from build123d import *

# Parameters (mm, degrees)
SKETCH_1_R        = 3.75
SKETCH_1_R_2      = 2.75
EXTRUDE_250_DEPTH = 4
EXTRUDE_START     = 4
SKETCH_2_R        = 1.7
SKETCH_2_R_2      = 2.75
EXTRUDE_354_DEPTH = 5


with BuildPart() as part:
    # 草图1 → Extrude 250 (new body)
    with BuildSketch(Plane.XY):
        Polygon((-55, -44), (-49, -50), (49, -50), (55, -44), (55, 44), (49, 50), (-49, 50), (-55, 44), (-55, 10), (12, 10), (12, -10), (-55, -10), align=None)
        with Locations((-14.845, -14.845)):
            Circle(SKETCH_1_R, mode=Mode.SUBTRACT)
        with Locations((-14.845, 14.845)):
            Circle(SKETCH_1_R, mode=Mode.SUBTRACT)
        with Locations((14.845, -14.845)):
            Circle(SKETCH_1_R, mode=Mode.SUBTRACT)
        with Locations((14.845, 14.845)):
            Circle(SKETCH_1_R, mode=Mode.SUBTRACT)
        with Locations((-44, -39)):
            Circle(SKETCH_1_R_2, mode=Mode.SUBTRACT)
        with Locations((-44, 39)):
            Circle(SKETCH_1_R_2, mode=Mode.SUBTRACT)
        with Locations((44, -39)):
            Circle(SKETCH_1_R_2, mode=Mode.SUBTRACT)
        with Locations((44, 39)):
            Circle(SKETCH_1_R_2, mode=Mode.SUBTRACT)
    extrude(amount=EXTRUDE_250_DEPTH)

    # 草图2 → Extrude 354 (add)
    with BuildSketch(Plane.XY.offset(EXTRUDE_START)):
        Polygon((-55, -44), (-49, -50), (49, -50), (55, -44), (55, 44), (49, 50), (-49, 50), (-55, 44), (-55, 10), (12, 10), (12, -10), (-55, -10), align=None)
        with Locations((-14.845, -14.845)):
            Circle(SKETCH_2_R, mode=Mode.SUBTRACT)
        with Locations((-14.845, 14.845)):
            Circle(SKETCH_2_R, mode=Mode.SUBTRACT)
        with Locations((14.845, -14.845)):
            Circle(SKETCH_2_R, mode=Mode.SUBTRACT)
        with Locations((14.845, 14.845)):
            Circle(SKETCH_2_R, mode=Mode.SUBTRACT)
        with Locations((-44, -39)):
            Circle(SKETCH_2_R_2, mode=Mode.SUBTRACT)
        with Locations((-44, 39)):
            Circle(SKETCH_2_R_2, mode=Mode.SUBTRACT)
        with Locations((44, -39)):
            Circle(SKETCH_2_R_2, mode=Mode.SUBTRACT)
        with Locations((44, 39)):
            Circle(SKETCH_2_R_2, mode=Mode.SUBTRACT)
    extrude(amount=EXTRUDE_354_DEPTH)


solid = part.part
For this review, take the finished solid that the model builds, in its own axes (mm). A direction names the side the tool comes from. Coordinates: 2 decimals unless noted, no trailing zeros. Order: outer loops, then holes, each group sorted by start corner. A loop starts at its lowest first (then second) coordinate and runs counter-clockwise, first axis right, second up. Notation, with made-up numbers: (71.5, 25) - (101.5, 25) arc R16 cw to (101.5, 53) - close; hole circle Ø5 at (56, 32.5). An arc over 180 degrees is marked (long way). Answer as CSV lines item,"result". Start each with the question number.
1) Add section B-B (x = 44). State the section outline as (y, z) points.
2) Draft analysis for pull direction Y (two halves, no side actions). For faces 4 (the flat face through (52, -47, 4)), 5 (the flat face through (55, -1, 4)), 6 (the cylindrical face through (-46.027, 40.859, 4.437)), state which applies: +Y half, -Y half, draft (parallel to the pull), parting line (faces both ways), or undercut.
3) Insertion check: P1, Ø5.5, axis at x = -14.845, y = 14.845, coming from the -Z side. The pin has a flat end and moves straight along its axis. Give the tip position at first contact, or say it passes through.
4) Add section D-D (x = -44). State the section outline as (y, z) points.
5) To check wall thickness, follow line 1 along Y through (x, z) = (-44, 4.5); line 2 along Y through (x, z) = (-41, 3.5); line 3 along Y through (x, z) = (44, 4.5). State the ranges of each line that lie inside material, in increasing order. Write a range as [from, to].
6) Machinability: for faces 1 (the cylindrical face through (-15.658, 11.184, 1.972)), 2 (the flat face through (12, 0, 4)), 3 (the cylindrical face through (-16.543, -14.77, 6.465)), which of the approach directions +Z, -Z, +X, -X, +Y, -Y give a long, thin tool a straight path to every point of the face, cutting with its end or side? Answer none if there is none.
7) Add section A-A (x = 6.5). State the section outline as (y, z) points, then the cut area to 3 significant figures.
8) Add section C-C (y = -39). State the section outline as (x, z) points, then the cut area to 3 significant figures.
Result:
1,outline,"(-50, 0) - (-41.75, 0) - (-41.75, 9) - (-50, 9) - close; (-36.25, 0) - (36.25, 0) - (36.25, 9) - (-36.25, 9) - close; (41.75, 0) - (50, 0) - (50, 9) - (41.75, 9) - close"
2,face 4,"-Y half"
2,face 5,"draft"
2,face 6,"undercut"
3,P1,"z = 4"
4,outline,"(-50, 0) - (-41.75, 0) - (-41.75, 9) - (-50, 9) - close; (-36.25, 0) - (-10, 0) - (-10, 9) - (-36.25, 9) - close; (10, 0) - (36.25, 0) - (36.25, 9) - (10, 9) - close; (41.75, 0) - (50, 0) - (50, 9) - (41.75, 9) - close"
5,line 1,"[-50, -41.75], [-36.25, -10], [10, 36.25], [41.75, 50]"
5,line 2,"[-50, -10], [10, 50]"
5,line 3,"[-50, -41.75], [-36.25, 36.25], [41.75, 50]"
6,face 1,"-Z"
6,face 2,"+Z, -Z, -X"
6,face 3,"+Z, -Z"
7,outline,"(-50, 0) - (-10, 0) - (-10, 9) - (-50, 9) - close; (10, 0) - (50, 0) - (50, 9) - (10, 9) - close"
7,area,"720 mm^2"
8,outline,"(-55, 0) - (-46.75, 0) - (-46.75, 9) - (-55, 9) - close; (-41.25, 0) - (41.25, 0) - (41.25, 9) - (-41.25, 9) - close; (46.75, 0) - (55, 0) - (55, 9) - (46.75, 9) - close"
8,area,"891 mm^2"
